from build123d import *

# Parameters (mm, degrees)
BOSS_EXTRUDE1_DEPTH      = 30
BOSS_EXTRUDE1_DEPTH_BACK = 30
SKETCH1_R                = 18
SKETCH1_R_2              = 6
CUT_EXTRUDE1_DEPTH       = 124.310147564
CUT_EXTRUDE2_DEPTH       = 124.310147564
CUT_EXTRUDE3_DEPTH       = 121.573628958


with BuildPart() as part:
    # Sketch1 → Boss-Extrude1 (new, two sides: drawn at the far end of the back side and taken through both)
    with BuildSketch(Plane(origin=(0, 0, 0), x_dir=(1, 0, 0), z_dir=(0, 1, 0)).offset(-BOSS_EXTRUDE1_DEPTH_BACK)):
        with BuildLine():
            Line((3.25, 24.787849846), (101.56, 11.898167926))
            ThreePointArc((101.56, 11.898167926), (112, 0), (101.56, -11.898167926))
            Line((101.56, -11.898167926), (3.25, -24.787849846))
            ThreePointArc((3.25, -24.787849846), (-25, 0), (3.25, 24.787849846))
        make_face()
        with Locations(Location((0, 0, 0), (0, 0, 270))):
            Circle(SKETCH1_R, mode=Mode.SUBTRACT)
        with Locations(Location((100, 0, 0), (0, 0, 270))):
            Circle(SKETCH1_R_2, mode=Mode.SUBTRACT)
        with BuildLine():
            Line((29.001639294, 14.62548865), (80.82543669, 8.361367746))
            ThreePointArc((80.82543669, 8.361367746), (88.001643881, 0.306494185), (80.906985676, -7.820298705))
            Line((80.906985676, -7.820298705), (29.051639294, -14.619189161))
            ThreePointArc((29.051639294, -14.619189161), (24.534716663, -12.831305196), (23.668032745, -8.051349326))
            ThreePointArc((23.668032745, -8.051349326), (25, 0), (23.668032745, 8.051349326))
            ThreePointArc((23.668032745, 8.051349326), (24.518792048, 12.811777483), (29.001639294, 14.62548865))
        make_face(mode=Mode.SUBTRACT)
    extrude(amount=BOSS_EXTRUDE1_DEPTH + BOSS_EXTRUDE1_DEPTH_BACK)

    # Sketch2 → Cut-Extrude1 (cut, through all)
    with BuildSketch(Plane(origin=(3.25, 0, 24.787849846), x_dir=(0.9915139938498094, 0, -0.1300000000000003), z_dir=(0.1300000000000003, 0, 0.9915139938498095))):
        Polygon((-25, 30), (-25, 7), (35, 7), (74.151399385, 30), align=None)
    cut_extrude1 = extrude(amount=-CUT_EXTRUDE1_DEPTH, mode=Mode.SUBTRACT)

    # Mirror1: Cut-Extrude1 across plane
    add(cut_extrude1.mirror(Plane.ZX), mode=Mode.SUBTRACT)

    # Sketch3 → Cut-Extrude2 (cut, through all)
    with BuildSketch(Plane(origin=(3.25, 0, 24.787849846), x_dir=(0.9915139938498094, 0, -0.1300000000000003), z_dir=(0.1300000000000003, 0, 0.9915139938498095))):
        with BuildLine():
            Line((111.151399385, -22), (111.151399385, 22))
            Line((111.151399385, 22), (74.151399385, 22))
            Line((74.151399385, 22), (54.046281618, 10.392304845))
            ThreePointArc((54.046281618, 10.392304845), (48.046281618, 0), (54.046281618, -10.392304845))
            Line((54.046281618, -10.392304845), (74.151399385, -22))
            Line((74.151399385, -22), (111.151399385, -22))
        make_face()
    extrude(amount=-CUT_EXTRUDE2_DEPTH, mode=Mode.SUBTRACT)

    # Sketch4 → Cut-Extrude3 (cut, through all)
    with BuildSketch(Plane(origin=(0, 7, 0), x_dir=(1, 0, 0), z_dir=(0, 1, 0))):
        with BuildLine():
            Line((8.691485355, 15.762553167), (12.227019261, 19.298087073))
            Line((12.227019261, 19.298087073), (19.298087073, 12.227019261))
            Line((19.298087073, 12.227019261), (15.762553167, 8.691485355))
            ThreePointArc((15.762553167, 8.691485355), (12.727922061, 12.727922061), (8.691485355, 15.762553167))
        make_face()
    extrude(amount=-CUT_EXTRUDE3_DEPTH, mode=Mode.SUBTRACT)


solid = part.part
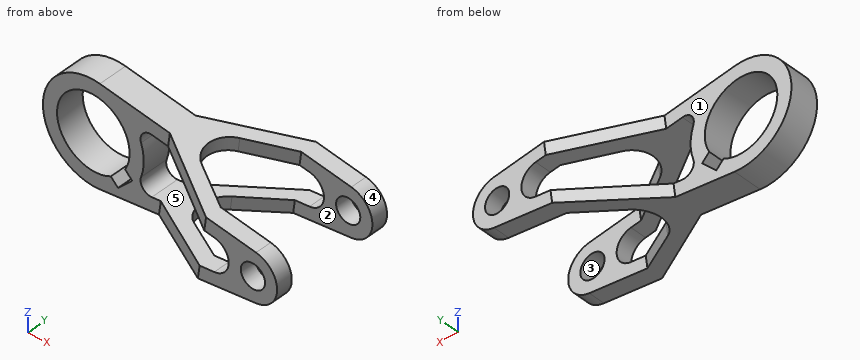
Design review of the part built by this model. Coordinates are the model's own, in mm. Face numbers are marked on the shaded views. A direction names the side the tool comes from. Round coordinates to 2 decimals unless told otherwise and drop trailing zeros. Loops run counter-clockwise (first coordinate to the right, second up) from the corner with the lowest first, then second, coordinate; pieces in that order, holes last. Notation, with made-up numbers: M -36.5,-25 L -25.5,-25 A12 ccw -25.5,-7 Z; hole C 39,34 d9. An arc over 180 degrees is marked long. Answer as a JSON object with one key per item and string values.
Item 1: The part is to be moulded in two halves that separate along Y. For the marked faces 1, 2 and 3, say which applies: pulls with the +Y half, pulls with the -Y half, needs draft (parallel to the pull), parting line crosses it, or undercut.
Answer sheet:
{"face 1": "pulls with the +Y half", "face 2": "undercut", "face 3": "needs draft"}
Item 2: Wall thickness on L1, parallel to Y at x = 78, z = 11; L2, parallel to Z at x = 0, y = 4; L3, parallel to Z at x = 100, y = 26: over which ranges is each line inside the solid? List them lowest first. Write a range as from..to.
Answer sheet:
{"L1": "y = -30..-22, 22..30", "L2": "z = -25..-18, 18..25", "L3": "z = -12.1..-6, 6..12.1"}
Item 3: We need section A-A on x = 0. Give the boundary of the cut face in (y, z).
Answer sheet:
{"outline": "M -7,-25 L 7,-25 L 7,-18 L -7,-18 Z; M -7,18 L 7,18 L 7,25 L -7,25 Z"}
Item 4: We need section C-C on y = -9. Give the boundary of the cut face in (x, z).
Answer sheet:
{"outline": "M 36.05,-20.49 L 50.11,-18.64 L 50.99,-11.97 L 36.94,-13.67 Z; M 40.45,13.12 L 54.04,11.34 L 54.92,18.01 L 41.33,19.8 Z"}
Item 5: We need section D-D on x = 100. Give the boundary of the cut face in (y, z).
Answer sheet:
{"outline": "M -30,-12.1 L -22,-12.1 L -22,-6 L -30,-6 Z; M -30,6 L -22,6 L -22,12.1 L -30,12.1 Z; M 22,-12.1 L 30,-12.1 L 30,-6 L 22,-6 Z; M 22,6 L 30,6 L 30,12.1 L 22,12.1 Z"}
Item 6: Machinability: for the marked faces 4 and 5, which of the approach directions +Z, -Z, +X, -X, +Y, -Y give a long, thin tool a straight path to every point of the face, cutting with its end or side? Answer none if there is none.
Answer sheet:
{"face 4": "+X, +Y, -Y", "face 5": "+Y, -Y"}
Item 7: We need section B-B on z = 1. Give the boundary of the cut face in (x, y).
Answer sheet:
{"outline": "M -24.98,-7 L -17.97,-7 L -17.97,7 L -24.98,7 Z; M 17.97,-7 L 24.98,-7 L 24.98,7 L 17.97,7 Z; M 87.9,-30 L 94.08,-30 L 94.08,-22 L 87.9,-22 Z; M 87.9,22 L 94.08,22 L 94.08,30 L 87.9,30 Z; M 105.92,-30 L 111.96,-30 L 111.96,-22 L 105.92,-22 Z; M 105.92,22 L 111.96,22 L 111.96,30 L 105.92,30 Z"}
Item 8: Clearance check with flat-ended pins moving along their axes: P1, Ø5, axis at y = -18, z = 16.5, coming from the +X side; P2, Ø2, axis at y = 23, z = -10, coming from the -X side; P3, Ø8, axis at x = 16, y = -1, coming from the +Z side. State where each tip first meets the part, or that it passes through.
Answer sheet:
{"P1": "stops at x = 73.86", "P2": "stops at x = 60.39", "P3": "stops at z = 23.64"}
